Study the drawing (mm; zero at the part's minimum x, y, z) and answer. Give positions to 0.01 mm unless a question says otherwise; leave off trailing zeros. Loops run counter-clockwise (first coordinate to the right, second up) from the corner with the lowest first, then second, coordinate; pieces in that order, holes last. Notation, with made-up numbers: (5, 0.25) - (47, 0.25) arc R22 cw to (47, 32.25) - close; hole circle Ø9 at (62, 80). An arc over 180 degrees is marked (long way). Answer in a Markdown table with one row per item. Add a question column.
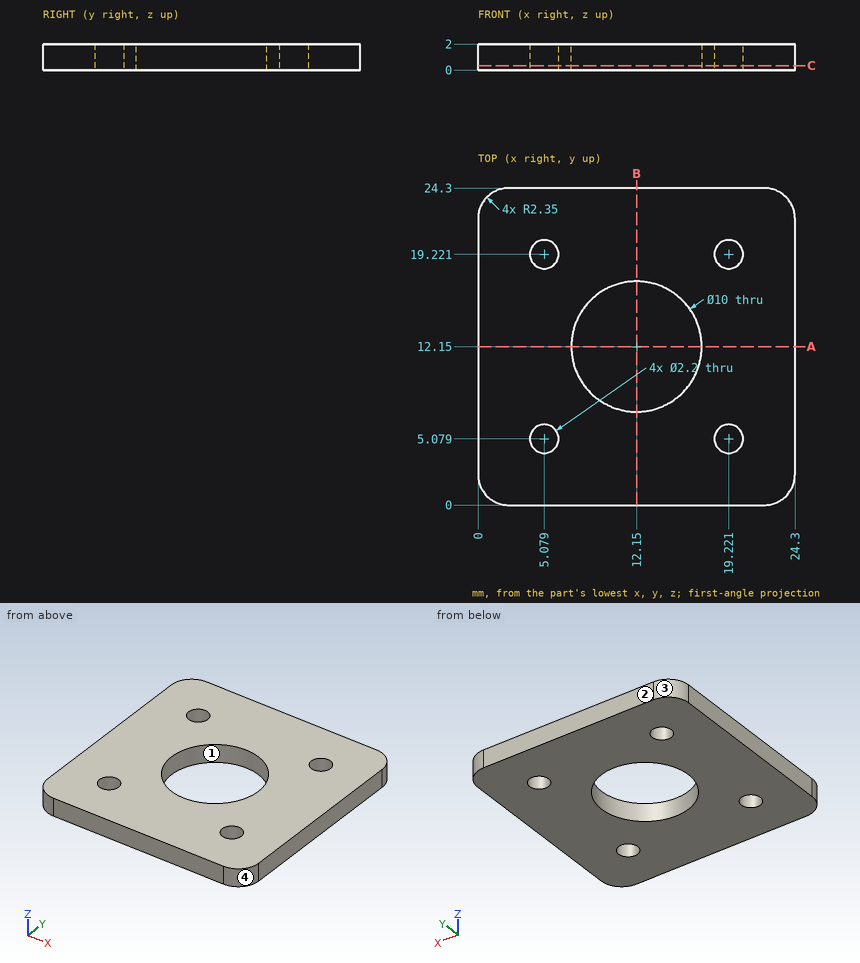
(1) Find the intervals of material crossed by line 1 along Y through (x, z) = (19, 1.75); line 2 along Y through (x, z) = (20, 1.85); line 3 along Y through (x, z) = (2.25, 0.2), in increasing order. Write a range as [from, to].
(2) A cutting plane is placed at A-A on y = 12.15. Determine the outline of the cut face in (x, z).
(3) A cutting plane is placed at C-C on z = 0.35. Determine the outline of the cut face in (x, y).
(4) The mould has two halves that part along X. Classify the marked faces 1, 2, 3 and 4: pulls with the +X half, pulls with the -X half, needs draft (parallel to the pull), parting line crosses it, or undercut.
Evaluation:
| question | item | result |
|---|---|---|
| 1 | line 1 | y = [0, 4], [6.16, 18.14], [20.3, 24.3] |
| 1 | line 2 | y = [0, 4.3], [5.86, 18.44], [20, 24.3] |
| 1 | line 3 | y = [0, 24.3] |
| 2 | outline | (0, 0) - (7.15, 0) - (7.15, 2) - (0, 2) - close; (17.15, 0) - (24.3, 0) - (24.3, 2) - (17.15, 2) - close |
| 3 | outline | (0, 2.35) arc R2.35 ccw to (2.35, 0) - (21.95, 0) arc R2.35 ccw to (24.3, 2.35) - (24.3, 21.95) arc R2.35 ccw to (21.95, 24.3) - (2.35, 24.3) arc R2.35 ccw to (0, 21.95) - close; hole circle Ø2.2 at (5.08, 5.08); hole circle Ø2.2 at (5.08, 19.22); hole circle Ø10 at (12.15, 12.15); hole circle Ø2.2 at (19.22, 5.08); hole circle Ø2.2 at (19.22, 19.22) |
| 4 | face 1 | undercut |
| 4 | face 2 | needs draft |
| 4 | face 3 | pulls with the -X half |
| 4 | face 4 | pulls with the +X half |
